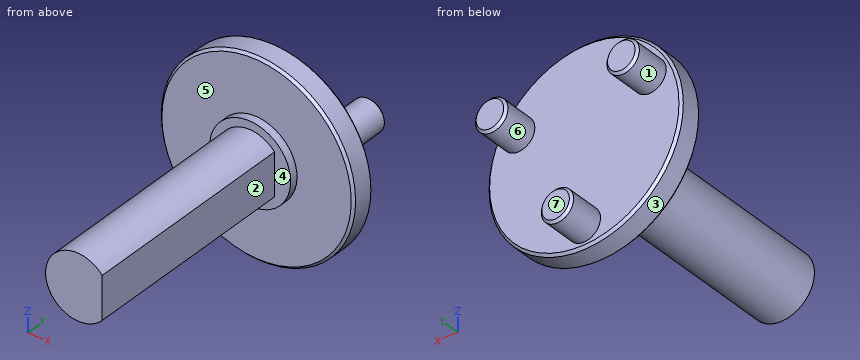
```python
from build123d import *

# Parameters (mm, degrees)
SKETCH1_R           = 12
BOSS_EXTRUDE1_DEPTH = 3
SKETCH2_R           = 2
BOSS_EXTRUDE2_DEPTH = 4.5
SKETCH3_R           = 5
BOSS_EXTRUDE3_DEPTH = 1
BOSS_EXTRUDE4_DEPTH = 27
CHAMFER1_SIZE       = 0.3


with BuildPart() as part:
    # Sketch1 → Boss-Extrude1 (new body)
    with BuildSketch(Plane(origin=(0, 0, 0), x_dir=(1, 0, 0), z_dir=(0, 1, 0))):
        with Locations(Location((0, 0, 0), (0, 0, 270))):
            Circle(SKETCH1_R)
    extrude(amount=BOSS_EXTRUDE1_DEPTH)

    # Sketch2 → Boss-Extrude2 (add)
    with BuildSketch(Plane(origin=(0, 3, 0), x_dir=(1, 0, 0), z_dir=(0, 1, 0))):
        with Locations(Location((0, 9.37, 0), (0, 0, 270))):
            Circle(SKETCH2_R)
        with Locations(Location((-8.114658033, -4.685, 0), (0, 0, 270))):
            Circle(SKETCH2_R)
        with Locations(Location((8.114658033, -4.685, 0), (0, 0, 270))):
            Circle(SKETCH2_R)
    extrude(amount=BOSS_EXTRUDE2_DEPTH)

    # Sketch3 → Boss-Extrude3 (add)
    with BuildSketch(Plane.XZ):
        with Locations(Location((0, 0, 0), (0, 0, 270))):
            Circle(SKETCH3_R)
    extrude(amount=BOSS_EXTRUDE3_DEPTH)

    # Sketch4 → Boss-Extrude4 (add)
    with BuildSketch(Plane.XZ.offset(1)):
        with BuildLine():
            Line((3, 2.645751311), (3, -2.645751311))
            ThreePointArc((3, -2.645751311), (-4, 0), (3, 2.645751311))
        make_face()
    extrude(amount=BOSS_EXTRUDE4_DEPTH)

    # Chamfer1
    chamfer1_edges = [part.edges().sort_by_distance(p)[0] for p in [
        (-8.114658033, 7.5, 2.685),
        (8.114658033, 7.5, 2.685),
        (0, 0, -12),
        (0, 3, -12),
        (0, 7.5, -11.37),
    ]]
    chamfer(chamfer1_edges, length=CHAMFER1_SIZE)


solid = part.part
```
Check sheet for the modelled part. Datum: model origin and axes. Units: mm. Face numbers are marked on the shaded views. A direction names the side the tool comes from. Round coordinates to 2 decimals unless told otherwise and drop trailing zeros. Loops run counter-clockwise (first coordinate to the right, second up) from the corner with the lowest first, then second, coordinate; pieces in that order, holes last. Notation, with made-up numbers: (0.5, -23) -> (28.5, -23) arc R21 ccw to (28.5, 1) -> close; hole circle Ø1 at (69, 3). An arc over 180 degrees is marked (long way). Answer in a Markdown table with one row per item.
Q1. Release check for a two-part mould opening along X. For the marked faces 1, 2, 3 and 4 record: released by +X, released by -X, zero draft, split by the parting line, or undercut.
Data:
| item | result |
|---|---|
| face 1 | undercut |
| face 2 | released by +X |
| face 3 | split by the parting line |
| face 4 | zero draft |
Q2. Sectioned sample at A-A on x = 0. Enter the section's corners in (y, z).
Data:
| item | result |
|---|---|
| outline | (-28, -4) -> (-1, -4) -> (-1, -5) -> (0, -5) -> (0, -11.7) -> (0.3, -12) -> (2.7, -12) -> (3, -11.7) -> (3, -11.37) -> (7.2, -11.37) -> (7.5, -11.07) -> (7.5, -7.67) -> (7.2, -7.37) -> (3, -7.37) -> (3, 11.7) -> (2.7, 12) -> (0.3, 12) -> (0, 11.7) -> (0, 5) -> (-1, 5) -> (-1, 4) -> (-28, 4) -> close |
Q3. Sectioned sample at B-B on z = 0. Enter the section's corners in (x, y).
Data:
| item | result |
|---|---|
| outline | (-12, 0.3) -> (-11.7, 0) -> (-5, 0) -> (-5, -1) -> (-4, -1) -> (-4, -28) -> (3, -28) -> (3, -1) -> (5, -1) -> (5, 0) -> (11.7, 0) -> (12, 0.3) -> (12, 2.7) -> (11.7, 3) -> (-11.7, 3) -> (-12, 2.7) -> close |
Q4. Go/stop test with flat-tipped pins: P1, Ø1.5, axis at y = 2, z = 1.5, coming from the -X side; P2, Ø12, axis at y = -0.5, z = -8.5, coming from the +X side; P3, Ø4, axis at x = -4, y = -13, coming from the +Z side; P4, Ø11.5, axis at x = -3, z = 0, coming from the +Y side. Record where each tip stops, or that it passes through.
Data:
| item | result |
|---|---|
| P1 | stops at x = -11.98 |
| P2 | stops at x = 11.73 |
| P3 | stops at z = 3.46 |
| P4 | stops at y = 7.5 |
Q5. Thickness scan on L1, parallel to Y at x = 4.5, z = -2.5; L2, parallel to Y at x = -9.5, z = 5.25; L3, parallel to X at y = -6.5, z = 1.25. Record the ranges inside material, lowest first.
Data:
| item | result |
|---|---|
| L1 | y = 0 to 3 |
| L2 | y = 0 to 7.5 |
| L3 | x = -3.8 to 3 |
Q6. Set-up check for the marked faces 5, 6 and 7: record each of +Z, -Z, +X, -X, +Y, -Y from which the full face is reachable in a straight line by a thin tool's end or side.
Data:
| item | result |
|---|---|
| face 5 | -Y |
| face 6 | +Y |
| face 7 | +Z, -Z, +X, -X, +Y |
Q7. Sectioned sample at C-C on y = -11.5. Enter the section's corners in (x, z).
Data:
| item | result |
|---|---|
| outline | (3, -2.65) -> (3, 2.65) arc R4 ccw (long way) to start |
